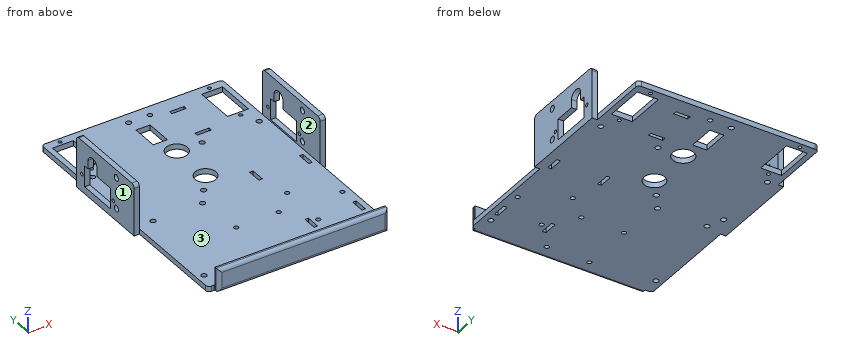
```python
from build123d import *

# Parameters (mm, degrees)
MODEL_R                  = 1.5
MODEL_R_2                = 1
MODEL_R_3                = 6
MODEL_R_4                = 1.25
MODEL_R_5                = 1.349782665
MODEL_R_6                = 5.9
MODEL_W                  = 8
MODEL_H                  = 15
MODEL_H_2                = 2
MODEL_W_2                = 11.8
MODEL_H_3                = 22.5
MODEL_W_3                = 2
MODEL_H_4                = 8
MODEL_H_5                = 7.999999999
SALIENTE_EXTRUIR1_DEPTH  = 3
CROQUIS2_W               = 3
CROQUIS2_H               = 50
SALIENTE_EXTRUIR2_DEPTH  = 29
CROQUIS3_R               = 1.765481919
CROQUIS3_R_2             = 1
CORTAR_EXTRUIR1_DEPTH    = 3
REDONDEO1_R              = 2
REDONDEO1_OF_SIMETR_A1_R = 2
CROQUIS4_W               = 96
CROQUIS4_H               = 3
SALIENTE_EXTRUIR3_DEPTH  = 13
REDONDEO2_R              = 2


with BuildPart() as part:
    # Model → Saliente-Extruir1 (new body)
    with BuildSketch(Plane.XY):
        with BuildLine():
            Line((13.198959583, -198.58599061), (108.142640241, -198.58599061))
            Line((108.142640241, -198.58599061), (109.670799912, -198.585990609))
            ThreePointArc((109.670799912, -198.585990609), (111.085013474, -198.000204172), (111.670799912, -196.58599061))
            Line((111.670799912, -196.58599061), (111.670799912, -139.134723681))
            Line((111.670799912, -139.134723681), (114.670799912, -139.134723681))
            Line((114.670799912, -139.134723681), (114.670799912, -89.134723681))
            Line((114.670799912, -89.134723681), (111.670799912, -89.134723681))
            Line((111.670799912, -89.134723681), (111.670799912, -56.020997464))
            ThreePointArc((111.670799912, -56.020997464), (111.085013474, -54.606783901), (109.670799912, -54.020997464))
            Line((109.670799912, -54.020997464), (77.898959582, -54.020997464))
            Line((77.898959582, -54.020997464), (43.555278924, -54.020997464))
            Line((43.555278924, -54.020997464), (11.670799912, -54.020997464))
            ThreePointArc((11.670799912, -54.020997464), (10.256586349, -54.606783901), (9.670799912, -56.020997464))
            Line((9.670799912, -56.020997464), (9.670799912, -89.134723681))
            Line((9.670799912, -89.134723681), (6.670799912, -89.134723681))
            Line((6.670799912, -89.134723681), (6.670799912, -139.134723681))
            Line((6.670799912, -139.134723681), (9.670799912, -139.134723681))
            Line((9.670799912, -139.134723681), (9.670799912, -196.585990609))
            ThreePointArc((9.670799912, -196.585990609), (10.256586349, -198.000204172), (11.670799912, -198.585990609))
            Line((11.670799912, -198.585990609), (13.198959583, -198.58599061))
        make_face()
        with Locations((107.170799912, -93.113896801)):
            Circle(MODEL_R, mode=Mode.SUBTRACT)
        with Locations((102.770799912, -56.620997464)):
            Circle(MODEL_R_2, mode=Mode.SUBTRACT)
        with Locations((102.770799912, -83.920997464)):
            Circle(MODEL_R_2, mode=Mode.SUBTRACT)
        with Locations((18.570799912, -83.920997464)):
            Circle(MODEL_R_2, mode=Mode.SUBTRACT)
        with Locations((18.570799912, -56.620997464)):
            Circle(MODEL_R_2, mode=Mode.SUBTRACT)
        with Locations((60.670799912, -93.098913634)):
            Circle(MODEL_R_3, mode=Mode.SUBTRACT)
        with Locations((15.170799912, -90.015990609)):
            Circle(MODEL_R, mode=Mode.SUBTRACT)
        with Locations((46.690799912, -137.01599061)):
            Circle(MODEL_R, mode=Mode.SUBTRACT)
        with Locations((18.750799912, -137.01599061)):
            Circle(MODEL_R, mode=Mode.SUBTRACT)
        with Locations((13.670799912, -189.085990609)):
            Circle(MODEL_R, mode=Mode.SUBTRACT)
        with Locations((53.170799912, -128.015990609)):
            Circle(MODEL_R, mode=Mode.SUBTRACT)
        with Locations((15.170799912, -128.015990609)):
            Circle(MODEL_R, mode=Mode.SUBTRACT)
        with Locations((107.373959583, -165.015945956)):
            Circle(MODEL_R_4, mode=Mode.SUBTRACT)
        with Locations((85.023959582, -151.515945956)):
            Circle(MODEL_R_4, mode=Mode.SUBTRACT)
        with Locations((85.023959582, -178.515945956)):
            Circle(MODEL_R_4, mode=Mode.SUBTRACT)
        with Locations((66.670799912, -60.520997464)):
            Circle(MODEL_R_5, mode=Mode.SUBTRACT)
        with Locations((107.170799912, -188.585990609)):
            Circle(MODEL_R, mode=Mode.SUBTRACT)
        with Locations((74.670799912, -93.580727597)):
            Circle(MODEL_R, mode=Mode.SUBTRACT)
        with Locations((60.670799912, -118.098913634)):
            Circle(MODEL_R_6, mode=Mode.SUBTRACT)
        with Locations((54.698959583, -60.520997464)):
            Circle(MODEL_R, mode=Mode.SUBTRACT)
        with Locations((48.698959583, -193.085990609)):
            Circle(MODEL_R_4, mode=Mode.SUBTRACT)
        with Locations((72.727119253, -193.085990609)):
            Circle(MODEL_R_4, mode=Mode.SUBTRACT)
        with Locations((72.698959582, -163.085990609)):
            Circle(MODEL_R_4, mode=Mode.SUBTRACT)
        with Locations((48.698959583, -163.085990609)):
            Circle(MODEL_R_4, mode=Mode.SUBTRACT)
        with Locations((58.198959582, -75.127025732)):
            Rectangle(MODEL_W, MODEL_H, mode=Mode.SUBTRACT)
        with Locations((80.198959582, -64.186772947)):
            Rectangle(MODEL_W, MODEL_H_2, mode=Mode.SUBTRACT)
        with Locations((80.198959582, -86.067481229)):
            Rectangle(MODEL_W, MODEL_H_2, mode=Mode.SUBTRACT)
        with Locations((102.770799912, -70.270997464)):
            Rectangle(MODEL_W_2, MODEL_H_3, mode=Mode.SUBTRACT)
        with Locations((18.570799912, -70.270997464)):
            Rectangle(MODEL_W_2, MODEL_H_3, mode=Mode.SUBTRACT)
        with Locations((80.698959582, -179.08599061)):
            Rectangle(MODEL_W_3, MODEL_H_4, mode=Mode.SUBTRACT)
        with Locations((107.670799912, -179.08599061)):
            Rectangle(MODEL_W_3, MODEL_H_5, mode=Mode.SUBTRACT)
        with Locations((80.698959582, -131.08599061)):
            Rectangle(MODEL_W_3, MODEL_H_4, mode=Mode.SUBTRACT)
        with Locations((108.198959582, -132.085990609)):
            Rectangle(MODEL_W_3, MODEL_H_4, mode=Mode.SUBTRACT)
    extrude(amount=SALIENTE_EXTRUIR1_DEPTH)

    # Croquis2 → Saliente-Extruir2 (add)
    with BuildSketch(Plane(origin=(0, 0, 0), x_dir=(-1, 0, 0), z_dir=(0, 0, -1))):
        with Locations((-113.170799912, -114.134723681)):
            Rectangle(CROQUIS2_W, CROQUIS2_H)
    saliente_extruir2 = extrude(amount=-SALIENTE_EXTRUIR2_DEPTH)

    # Croquis3 → Cortar-Extruir1 (cut)
    with BuildSketch(Plane(origin=(114.670799912, 0, 0), x_dir=(0, 0, -1), z_dir=(1, 0, 0))):
        with Locations((-24.5, -123.734723681)):
            Circle(CROQUIS3_R)
        with Locations((-7, -123.734723681)):
            Circle(CROQUIS3_R)
        with Locations((-9.9, -121.034548102)):
            Circle(CROQUIS3_R_2)
        with Locations((-9.9, -93.734723681)):
            Circle(CROQUIS3_R_2)
        with BuildLine():
            Line((-4, -118.634723681), (-4, -96.134723681))
            Line((-4, -96.134723681), (-15.8, -96.134723681))
            Line((-15.8, -96.134723681), (-15.8, -99.134723681))
            Line((-15.8, -99.134723681), (-20.577507922, -99.134723681))
            ThreePointArc((-20.577507922, -99.134723681), (-23.938367399, -103.128314954), (-20.488619892, -107.045378882))
            Line((-20.488619892, -107.045378882), (-15.8, -107.045378882))
            Line((-15.8, -107.045378882), (-15.8, -118.634723681))
            Line((-15.8, -118.634723681), (-4, -118.634723681))
        make_face()
    cortar_extruir1 = extrude(amount=-CORTAR_EXTRUIR1_DEPTH, mode=Mode.SUBTRACT)

    # Redondeo1
    redondeo1_edges = [part.edges().sort_by_distance(p)[0] for p in [
        (113.170799912, -89.134723681, 29),
        (113.170799912, -139.134723681, 29),
    ]]
    fillet(redondeo1_edges, radius=REDONDEO1_R)

    # Simetría1: Saliente-Extruir2, Cortar-Extruir1 across plane
    add(saliente_extruir2.mirror(Plane(origin=(60.670799912, 0, 0), x_dir=(0, 0, 1), z_dir=(1, 0, 0))))
    add(cortar_extruir1.mirror(Plane(origin=(60.670799912, 0, 0), x_dir=(0, 0, 1), z_dir=(1, 0, 0))), mode=Mode.SUBTRACT)

    # Redondeo1 of Simetría1
    redondeo1_of_simetr_a1_edges = [part.edges().sort_by_distance(p)[0] for p in [
        (8.170799912, -89.134723681, 29),
        (8.170799912, -139.134723681, 29),
    ]]
    fillet(redondeo1_of_simetr_a1_edges, radius=REDONDEO1_OF_SIMETR_A1_R)

    # Croquis4 → Saliente-Extruir3 (add)
    with BuildSketch(Plane(origin=(0, 0, 0), x_dir=(-1, 0, 0), z_dir=(0, 0, -1))):
        with Locations((-61.670799912, -200.085990609)):
            Rectangle(CROQUIS4_W, CROQUIS4_H)
    extrude(amount=-SALIENTE_EXTRUIR3_DEPTH)

    # Redondeo2
    redondeo2_edges = [part.edges().sort_by_distance(p)[0] for p in [
        (61.670799912, -201.585990609, 13),
        (13.670799912, -201.585990609, 6.5),
        (109.670799912, -201.585990609, 6.5),
        (61.670799912, -201.585990609, 0),
    ]]
    fillet(redondeo2_edges, radius=REDONDEO2_R)


solid = part.part
```
Source: CAD feature listing. Evaluate the final solid. Frame: model axes, mm. Face numbers are marked on the shaded views. A direction names the side the tool comes from. Give positions to 0.01 mm unless a question says otherwise; leave off trailing zeros. Loops run counter-clockwise (first coordinate to the right, second up) from the corner with the lowest first, then second, coordinate; pieces in that order, holes last. Notation, with made-up numbers: (45, 52) - (51, 52) arc R23 ccw to (51, 72) - close; hole circle Ø10 at (-25.5, 27). An arc over 180 degrees is marked (long way). Use CSV: the item, a comma, the result in double quotes. Start each with the question number.
1. Section B-B (y = -109). Output: boundary loops of the cut face in (x, z), then the cut area to 3 significant figures.
2. Pin query (flat end, axial travel): pin 1 (3.5 mm diameter, centred on x = 113.5, z = 19, fed in from -Y); pin 2 (0.9 mm diameter, centred on y = -179, z = 1.5, fed in from -X); pin 3 (1.5 mm diameter, centred on y = -78, z = 2, fed in from +X); pin 4 (2.5 mm diameter, centred on x = 15.17, y = -128.02, fed in from -Z). Return the tip coordinate at first contact, or that it passes through.
3. Ray query, L1, parallel to Y at x = 112.45, z = 7; L2, parallel to Y at x = 7.8, z = 24.5; L3, parallel to X at y = -130.5, z = 27.75. Return the intervals inside material, ascending.
4. Section C-C (y = -79.5). Output: boundary loops of the cut face in (x, z), then the cut area to 3 significant figures.
5. Section A-A (z = 7). Count the separate pieces of the cut face and the enclosed holes in it, then the cut area to 3 significant figures.
6. Reachability of the marked faces 1, 2 and 3 from +Z, -Z, +X, -X, +Y, -Y: full face, straight path, thin tool, end or side. Return the list, or none.
7. Section D-D (y = -172.5). Output: boundary loops of the cut face in (x, z), then the cut area to 3 significant figures.
Response:
1,outline,"(6.67, 0) - (114.67, 0) - (114.67, 4) - (111.67, 4) - (111.67, 3) - (9.67, 3) - (9.67, 4) - (6.67, 4) - close; (6.67, 15.8) - (9.67, 15.8) - (9.67, 29) - (6.67, 29) - close; (111.67, 15.8) - (114.67, 15.8) - (114.67, 29) - (111.67, 29) - close"
1,area,"409 mm²"
2,pin 1,"y = -139.13"
2,pin 2,"x = 9.67"
2,pin 3,"x = 111.67"
2,pin 4,"through"
3,L1,"-139.13 to -125.5, -121.97 to -118.63, -96.13 to -89.13"
3,L2,"-139.13 to -125.5, -121.97 to -89.13"
3,L3,"6.67 to 9.67, 111.67 to 114.67"
4,outline,"(9.67, 0) - (12.67, 0) - (12.67, 3) - (9.67, 3) - close; (24.47, 0) - (54.2, 0) - (54.2, 3) - (24.47, 3) - close; (62.2, 0) - (96.87, 0) - (96.87, 3) - (62.2, 3) - close; (108.67, 0) - (111.67, 0) - (111.67, 3) - (108.67, 3) - close"
4,area,"211 mm²"
5,separate pieces,"7"
5,enclosed holes,"0"
5,area,"430 mm²"
6,face 1,"+Z, -Z, -X, +Y, -Y"
6,face 2,"+Z, +Y, -Y"
6,face 3,"+Z, +Y"
7,outline,"(9.67, 0) - (111.67, 0) - (111.67, 3) - (9.67, 3) - close"
7,area,"306 mm²"
